from build123d import *

# Parameters (mm, degrees)
SKETCH_1_W          = 31.4
SKETCH_1_H          = 31.4
SKETCH_1_W_2        = 25
SKETCH_1_H_2        = 25
EXTRUDE_1_DEPTH     = 70
SKETCH_2_W          = 31.4
SKETCH_2_H          = 31.4
SKETCH_2_W_2        = 25
SKETCH_2_H_2        = 25
EXTRUDE_2_DEPTH     = 40
CUT_EXTRUDE_1_REACH = 84.137
SKETCH_3_W          = 25
SKETCH_3_H          = 25
FILLET_1_R          = 20
SKETCH_4_R          = 2.2
CUT_EXTRUDE_2_DEPTH = 95.807436417


with BuildPart() as part:
    # Эскиз1 → Вытянуть-Тонкостенный1 (new body)
    with BuildSketch(Plane(origin=(0, 0, 0), x_dir=(0, 0, -1), z_dir=(1, 0, 0))):
        Rectangle(SKETCH_1_W, SKETCH_1_H)
        Rectangle(SKETCH_1_W_2, SKETCH_1_H_2, mode=Mode.SUBTRACT)
    extrude(amount=EXTRUDE_1_DEPTH)

    # Эскиз2 → Вытянуть-Тонкостенный2 (add)
    with BuildSketch(Plane.XY.offset(15.7)):
        with Locations((35, 0)):
            Rectangle(SKETCH_2_W, SKETCH_2_H)
        with Locations((35, 0)):
            Rectangle(SKETCH_2_W_2, SKETCH_2_H_2, mode=Mode.SUBTRACT)
    extrude(amount=EXTRUDE_2_DEPTH)

    # Эскиз3 → Вырез-Вытянуть1 (cut, up to next)
    with BuildSketch(Plane.XY.offset(15.7), mode=Mode.PRIVATE) as cut_extrude_1_sk1:
        with Locations((35, 0)):
            Rectangle(SKETCH_3_W, SKETCH_3_H)
    cut_extrude_1_tool1 = extrude(cut_extrude_1_sk1.sketch, amount=-CUT_EXTRUDE_1_REACH, mode=Mode.PRIVATE) & part.part
    add(cut_extrude_1_tool1.solids().sort_by_distance((35, 0, 15.7))[0], mode=Mode.SUBTRACT)

    # Скругление1
    # the kernel refuses this fillet: 20 mm, written as the material it adds along each edge
    with BuildSketch(Plane(origin=(50.7, 15.7, 15.7), x_dir=(0, 0, 1), z_dir=(0, -1, 0))) as fillet_1_piece_1:
        with BuildLine():
            CenterArc((19.987746246, -20), FILLET_1_R, 90, 87.994238065)
            Line((0, -19.3), (-0.399754925, -19.286))
            ThreePointArc((-0.399754925, -19.286), (-0.4, -9.65), (-0.4, 0))
            Line((-0.4, 0), (0, 0.4))
            Line((0, 0.4), (19.987746246, 0.4))
            Line((19.987746246, 0.4), (19.987746246, 0))
        make_face()
    extrude(amount=31.4)
    with BuildSketch(Plane(origin=(19.3, -15.7, 15.7), x_dir=(-1, 0, 0), z_dir=(0, 1, 0))) as fillet_1_piece_2:
        with BuildLine():
            CenterArc((20, 19.987746246), FILLET_1_R, 180, 87.994238065)
            Line((0, 19.987746246), (-0.4, 19.987746246))
            Line((-0.4, 19.987746246), (-0.4, 0))
            Line((-0.4, 0), (0, -0.4))
            ThreePointArc((0, -0.4), (9.65, -0.4), (19.286, -0.399754925))
            Line((19.286, -0.399754925), (19.3, 0))
        make_face()
    extrude(amount=31.4)

    # Эскиз4 → Вырез-Вытянуть2 (cut, through all)
    with BuildSketch(Plane(origin=(0, 15.7, 0), x_dir=(1, 0, 0), z_dir=(0, 1, 0))):
        with Locations(Location((10, 0, 0), (0, 0, 270))):
            Circle(SKETCH_4_R)
        with Locations(Location((60, 0, 0), (0, 0, 270))):
            Circle(SKETCH_4_R)
        with Locations(Location((35, -45.7, 0), (0, 0, 270))):
            Circle(SKETCH_4_R)
        with Locations(Location((35, -20.7, 0), (0, 0, 270))):
            Circle(SKETCH_4_R)
    extrude(amount=-CUT_EXTRUDE_2_DEPTH, mode=Mode.SUBTRACT)


solid = part.part
Here's how the part is built. I have some questions about the finished solid (model axes, mm). A direction names the side the tool comes from. Coordinates: 2 decimals unless noted, no trailing zeros. Write each loop counter-clockwise with the first axis right and the second up, starting at its lowest first coordinate (ties: lowest second). Pieces come first, ordered by that corner, then holes.
Item 1: I want a section at B-B on y = -11. Write out the boundary of the cut face in (x, z), and give its area (3 significant figures).
Item 2: If we mould it in two halves opening along Z, with no side actions, what happens to faces 4 (the flat face through (11, 0, 12.5)), 5 (the flat face through (35, 15.7, 13)), 6 (the cylindrical face through (13.836, -0.22, 21.951))? For each: +Z half, -Z half, draft (parallel to the pull), parting line (faces both ways), or undercut.
Item 3: On a 3-axis mill with a long thin cutter (end or side, diameter ignored), from which of +Z, -Z, +X, -X, +Y, -Y can I reach the whole of each face in a straight line? I mean faces 1 (the flat face through (35, 12.5, 14)), 2 (the flat face through (35, 0, -12.5)), 3 (the flat face through (22.5, 0, 34)). Say none if no direction works.
Item 4: I want a section at D-D on z = 45.7. Write out the boundary of the cut face in (x, y), and give its area (3 significant figures).
Item 5: Will these pins go through, and if not, where does the flat tip stop? pin 1 (7.5 mm diameter, centred on y = 5, z = 26.5, fed in from +X); pin 2 (7.5 mm diameter, centred on y = -1.5, z = 41, fed in from -X); pin 3 (5 mm diameter, centred on x = 9, y = -4.5, fed in from +Z).
Item 6: If I drill on line 1 (X direction, y = 8, z = 51); line 2 (Y direction, x = 30, z = 19.5); line 3 (X direction, y = 13.45, z = 0), over which ranges is the centre line in solid material (lowest first)?
Item 7: I want a section at C-C on z = 0. Write out the boundary of the cut face in (x, y).
Item 8: I want a section at A-A on x = 35. Write out the boundary of the cut face in (y, z).
Findings below:
1. outline: (0, -15.7) - (70, -15.7) - (70, -12.5) - (0, -12.5) - close; (0, 12.5) - (22.5, 12.5) - (22.5, 55.7) - (19.3, 55.7) - (19.3, 35.69) arc R20 cw to (0, 15.7) - close; (47.5, 12.5) - (70, 12.5) - (70, 15.7) arc R20 cw to (50.7, 35.69) - (50.7, 55.7) - (47.5, 55.7) - close
1. area: 795 mm2
2. face 4: undercut
2. face 5: draft
2. face 6: +Z half
3. face 1: none
3. face 2: +X, -X
3. face 3: +Z
4. outline: (19.3, -15.7) - (32.8, -15.7) - (32.8, -12.5) - (22.5, -12.5) - (22.5, 12.5) - (32.8, 12.5) - (32.8, 15.7) - (19.3, 15.7) - close; (37.2, -15.7) - (50.7, -15.7) - (50.7, 15.7) - (37.2, 15.7) - (37.2, 12.5) - (47.5, 12.5) - (47.5, -12.5) - (37.2, -12.5) - close
4. area: 333 mm2
5. pin 1: stops at x = 55.45
5. pin 2: stops at x = 19.3
5. pin 3: stops at z = 19.84
6. line 1: x = 19.3 to 22.5, 47.5 to 50.7
6. line 2: y = -15.7 to -12.5, 12.5 to 15.7
6. line 3: x = 0 to 7.8, 12.2 to 57.8, 62.2 to 70
7. outline: (0, -15.7) - (7.8, -15.7) - (7.8, -12.5) - (0, -12.5) - close; (0, 12.5) - (7.8, 12.5) - (7.8, 15.7) - (0, 15.7) - close; (12.2, -15.7) - (57.8, -15.7) - (57.8, -12.5) - (12.2, -12.5) - close; (12.2, 12.5) - (57.8, 12.5) - (57.8, 15.7) - (12.2, 15.7) - close; (62.2, -15.7) - (70, -15.7) - (70, -12.5) - (62.2, -12.5) - close; (62.2, 12.5) - (70, 12.5) - (70, 15.7) - (62.2, 15.7) - close
8. outline: (-15.7, -15.7) - (15.7, -15.7) - (15.7, 18.5) - (12.5, 18.5) - (12.5, -12.5) - (-12.5, -12.5) - (-12.5, 18.5) - (-15.7, 18.5) - close; (-15.7, 22.9) - (-12.5, 22.9) - (-12.5, 43.5) - (-15.7, 43.5) - close; (-15.7, 47.9) - (-12.5, 47.9) - (-12.5, 55.7) - (-15.7, 55.7) - close; (12.5, 22.9) - (15.7, 22.9) - (15.7, 43.5) - (12.5, 43.5) - close; (12.5, 47.9) - (15.7, 47.9) - (15.7, 55.7) - (12.5, 55.7) - close
